CAD build for the part. Positions are in the model's coordinates, mm. A direction names the side the tool comes from. Coordinates: 2 decimals unless noted, no trailing zeros. Write each loop counter-clockwise with the first axis right and the second up, starting at its lowest first coordinate (ties: lowest second). Pieces come first, ordered by that corner, then holes. Notation, with made-up numbers: (36.5, 60) - (49.5, 60) arc R22 cw to (49.5, 91) - close; hole circle Ø1 at (75.5, -9). An arc over 180 degrees is marked (long way). Answer in a Markdown table with one row per item. Add a question column.
Q1. Drill centre lines: line 1 along X through (y, z) = (-3.5, 11.5); line 2 along Z through (x, y) = (41.5, -5.25); line 3 along X through (y, z) = (-4, 100). Where is each one in solid material? Low to high. Write a range as from..to.
Q2. Two-plate mould, pull along X, no slides. Class faces 1 (the flat face through (6, -6, 69)), 2 (the flat face through (65.621, -3, 13)), 3 (the cylindrical face through (55.555, -2.958, 24.462)): +X half, -X half, draft (parallel to the pull), parting line (faces both ways), or undercut.
Q3. Band-saw the part on B-B (x = -12.5). List the corners of the cut face in (y, z), and give its area (3 significant figures).
Q4. Pin check, flat tips, straight feed: pin 1 (1 mm diameter, centred on x = -6.5, y = -4, fed in from +Z); pin 2 (1 mm diameter, centred on x = -35, y = -2.5, fed in from -Z); pin 3 (1 mm diameter, centred on x = 4.5, y = -5, fed in from +Z). Stop position of each tip, or through.
Q5. 3-axis set-ups, long thin cutter, end or side, ignore diameter. For faces 4 (the flat face through (-5.36, -2.96, 59.23)), 5 (the cylindrical face through (-38.166, -2.958, 118.316)): which of +Z, -Z, +X, -X, +Y, -Y reach the whole face in a straight line?
Q6. Band-saw the part on C-C (z = 71). List the corners of the cut face in (x, y), and give its area (3 significant figures).
Q7. Band-saw the part on A-A (y = -3.7). List the corners of the cut face in (x, z).
```python
from build123d import *

# Parameters (mm, degrees)
F1_DEPTH = 6


with BuildPart() as f1:
    # F0 (on Front) → F1 (new body)
    with BuildSketch(Plane.XZ):
        Polygon((65.621033, -11.750089), (65.621033, 38.249911), (-24.378967, 128.249911), (-74.378967, 128.249911), align=None)
        with BuildLine():
            ThreePointArc((52.621032, 21.463115), (55.621032, 24.463115), (58.621032, 21.463115))
            Line((58.621032, 21.463115), (58.621032, 19.463115))
            ThreePointArc((58.621032, 19.463115), (55.621032, 16.463115), (52.621032, 19.463115))
            Line((52.621032, 19.463115), (52.621032, 21.463115))
        make_face(mode=Mode.SUBTRACT)
        with BuildLine():
            Line((-41.165764, 115.249911), (-43.165764, 115.249911))
            ThreePointArc((-43.165764, 115.249911), (-46.165764, 118.249911), (-43.165764, 121.249911))
            Line((-43.165764, 121.249911), (-41.165764, 121.249911))
            ThreePointArc((-41.165764, 121.249911), (-38.165764, 118.249911), (-41.165764, 115.249911))
        make_face(mode=Mode.SUBTRACT)
    extrude(amount=F1_DEPTH)


solid = f1.part
```
Checked values:
| question | item | result |
|---|---|---|
| 1 | line 1 | x = 42.37..65.62 |
| 1 | line 2 | z = 12.37..62.37 |
| 1 | line 3 | x = -46.13..3.87 |
| 2 | face 1 | draft |
| 2 | face 2 | +X half |
| 2 | face 3 | undercut |
| 3 | outline | (-6, 66.37) - (0, 66.37) - (0, 116.37) - (-6, 116.37) - close |
| 3 | area | 300 mm² |
| 4 | pin 1 | stops at z = 110.87 |
| 4 | pin 2 | stops at z = 88.37 |
| 4 | pin 3 | stops at z = 99.87 |
| 5 | face 4 | -Z, -X, +Y, -Y |
| 5 | face 5 | +Y, -Y |
| 6 | outline | (-17.13, -6) - (32.87, -6) - (32.87, 0) - (-17.13, 0) - close |
| 6 | area | 300 mm² |
| 7 | outline | (-74.38, 128.25) - (65.62, -11.75) - (65.62, 38.25) - (-24.38, 128.25) - close; hole (-43.17, 115.25) - (-41.17, 115.25) arc R3 ccw to (-41.17, 121.25) - (-43.17, 121.25) arc R3 ccw to start; hole (52.62, 19.46) arc R3 ccw to (58.62, 19.46) - (58.62, 21.46) arc R3 ccw to (52.62, 21.46) - close |
